Check sheet for the modelled part. Datum: model origin and axes. Units: mm. Round coordinates to 2 decimals unless told otherwise and drop trailing zeros. Write each loop counter-clockwise with the first axis right and the second up, starting at its lowest first coordinate (ties: lowest second). Pieces come first, ordered by that corner, then holes. Notation, with made-up numbers: (-10.5, 71) -> (7.5, 71) arc R3 ccw to (7.5, 75) -> close; hole circle Ø1 at (58, 24). An arc over 180 degrees is marked (long way). One line per item, written item: value.
from build123d import *

# Parameters (mm, degrees)
SKETCH1_R           = 250
BOSS_EXTRUDE1_DEPTH = 4
SKETCH5_R           = 2
CUT_EXTRUDE3_DEPTH  = 10


with BuildPart() as part:
    # Sketch1 → Boss-Extrude1 (new body)
    with BuildSketch(Plane.XY):
        Circle(SKETCH1_R)
    extrude(amount=BOSS_EXTRUDE1_DEPTH)

    # Sketch5 → Cut-Extrude3 (cut)
    with BuildSketch(Plane.XY.offset(4)):
        with Locations((-101.990381057, 146.652521874)):
            Circle(SKETCH5_R)
        with Locations((-76.009618943, 161.652521874)):
            Circle(SKETCH5_R)
        with Locations((-113.990381057, 167.437131564)):
            Circle(SKETCH5_R)
        with Locations((-88.009618943, 182.437131564)):
            Circle(SKETCH5_R)
        with Locations((76.009618943, 161.652521874)):
            Circle(SKETCH5_R)
        with Locations((101.990381057, 146.652521874)):
            Circle(SKETCH5_R)
        with Locations((88.009618943, 182.437131564)):
            Circle(SKETCH5_R)
        with Locations((113.990381057, 167.437131564)):
            Circle(SKETCH5_R)
        with Locations((101.990381057, -146.652521874)):
            Circle(SKETCH5_R)
        with Locations((76.009618943, -161.652521874)):
            Circle(SKETCH5_R)
        with Locations((113.990381057, -167.437131564)):
            Circle(SKETCH5_R)
        with Locations((88.009618943, -182.437131564)):
            Circle(SKETCH5_R)
        with Locations((-76.009618943, -161.652521874)):
            Circle(SKETCH5_R)
        with Locations((-101.990381057, -146.652521874)):
            Circle(SKETCH5_R)
        with Locations((-88.009618943, -182.437131564)):
            Circle(SKETCH5_R)
        with Locations((-113.990381057, -167.437131564)):
            Circle(SKETCH5_R)
    extrude(amount=-CUT_EXTRUDE3_DEPTH, mode=Mode.SUBTRACT)


solid = part.part
Item 1: Depth check by flat-ended pin: pin 1 (2 mm diameter, centred on y = 198.5, z = 3.5, fed in from +X); pin 2 (1 mm diameter, centred on x = 127, z = 1, fed in from -Y); pin 3 (1 mm diameter, centred on x = 133, z = 2, fed in from +Y). Enter the tip coordinate at first touch or a pass-through.
Result set:
pin 1: x = 153.28
pin 2: y = -215.63
pin 3: y = 212
Item 2: Sectioned sample at C-C (x = 60.5). Enter the section's corners in (y, z), then the cut area to 3 significant figures.
Result set:
outline: (-242.57, 0) -> (242.57, 0) -> (242.57, 4) -> (-242.57, 4) -> close
area: 1,940 mm^2
Item 3: Material ranges on line 1 along X through (y, z) = (147, 1.1); line 2 along X through (y, z) = (183, 2.5); line 3 along Y through (x, z) = (-5.5, 0.7), recorded low to high.
Result set:
line 1: -202.22 to -103.96, -100.02 to 100.02, 103.96 to 202.22
line 2: -170.33 to -89.93, -86.09 to 86.09, 89.93 to 170.33
line 3: -249.94 to 249.94
Item 4: Sectioned sample at B-B (y = -110). Enter the section's corners in (x, z).
Result set:
outline: (-224.5, 0) -> (224.5, 0) -> (224.5, 4) -> (-224.5, 4) -> close
Item 5: Sectioned sample at A-A (z = 1.45). State how many separate pieces and enclosed holes the cut face has, then the cut area to 3 significant figures.
Result set:
separate pieces: 1
enclosed holes: 16
area: 196,000 mm^2
